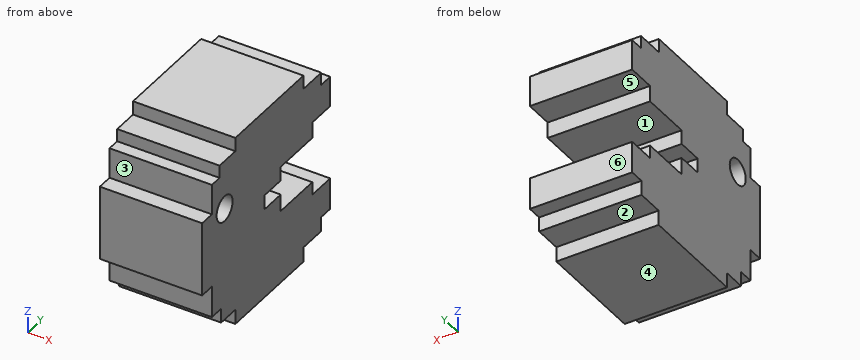
from build123d import *

# Parameters (mm, degrees)
F0_W     = 25.4
F0_H     = 25.399998
F1_DEPTH = 12.7
F3_DEPTH = 25.4
F4_R     = 1.5875
F5_DEPTH = 12.7


with BuildPart() as f1:
    # F0 (on Right) → F1 (new body)
    with BuildSketch(Plane.YZ):
        with Locations((12.7, 12.699999)):
            Rectangle(F0_W, F0_H)
    extrude(amount=F1_DEPTH)

    # F2 (on face) → F3 (cut)
    with BuildSketch(Plane.YZ.offset(12.7)):
        Polygon((0, 25.399998), (0, 16.820697), (1.931377, 16.820697), (1.931377, 20.601515), (3.452925, 20.601515), (3.452925, 22.169169), (6.588236, 22.169169), (6.588236, 23.875147), (20.09774, 23.875147), (20.09774, 22.169169), (23.624913, 22.169169), (23.624913, 20.601515), (25.4, 20.601515), (25.4, 25.399998), align=None)
        Polygon((0, 0), (6.588236, 0), (6.588236, 1.835753), (3.775678, 1.835753), (3.775678, 3.633947), (1.931377, 3.633947), (1.931377, 7.553086), (0, 7.553086), align=None)
        Polygon((20.143846, 1.835753), (20.143846, 0), (25.4, 0), (25.4, 3.633947), (23.555804, 3.633947), (23.555804, 1.835753), align=None)
        Polygon((21.849825, 7.553086), (25.4, 7.553086), (25.4, 16.820697), (21.849825, 16.820697), (21.849825, 14.838074), (15.579202, 14.838074), (15.579202, 13.085988), (12.397784, 13.085988), (12.397784, 11.287794), (15.579202, 11.287794), (15.579202, 9.166849), (21.849825, 9.166849), align=None)
    extrude(amount=-F3_DEPTH, mode=Mode.SUBTRACT)

    # F4 (on face) → F5 (cut)
    with BuildSketch(Plane.YZ.offset(12.7)):
        with Locations((4.452611, 16.06866)):
            Circle(F4_R)
    extrude(amount=-F5_DEPTH, mode=Mode.SUBTRACT)


solid = f1.part
Verification items for the finished model (mm, model axes). Face numbers are marked on the shaded views. A direction names the side the tool comes from. Coordinates: 2 decimals unless noted, no trailing zeros. Loops run counter-clockwise (first coordinate to the right, second up) from the corner with the lowest first, then second, coordinate; pieces in that order, holes last. Notation, with made-up numbers: (48, 41.25) -> (73, 41.25) arc R19 ccw to (73, 47.25) -> close; hole circle Ø8 at (7, -22.75). An arc over 180 degrees is marked (long way). Answer as a JSON object with one key per item and string values. Group by question number.
Item 1: Tool access check on the marked faces 1, 2 and 3. Record the directions out of +Z, -Z, +X, -X, +Y, -Y that give a thin tool (end or side, any length) a straight path to the whole face; none if there is none.
Item 2: Mould release check, pull along Z, two halves, no side actions. Record for the marked faces 4, 5 and 6: +Z half, -Z half, draft (parallel to the pull), parting line (faces both ways), or undercut.
Item 3: Scan lines: probe 1 along Z at (x, y) = (4.25, 23); probe 2 along Z at (x, y) = (10.75, 24); probe 3 along Y at (x, z) = (8.5, 1.5). Record each from-to range of solid material in increasing order.
Item 4: Sectioned sample at A-A on y = 18.75. Record the boundary of the cut face in (x, z).
Item 5: Sectioned sample at C-C on y = 14.5. Record the boundary of the cut face in (x, z).
Item 6: Depth check by flat-ended pin: pin 1 (2 mm diameter, centred on x = 3, z = 1, fed in from +Y); pin 2 (7 mm diameter, centred on x = 3, y = 19.5, fed in from -Z); pin 3 (1.9 mm diameter, centred on x = 5, z = 18, fed in from -Y); pin 4 (2 mm diameter, centred on x = 9.5, y = 1.5, fed in from -Z). Enter the tip coordinate at first touch or a pass-through.
Item 7: Sectioned sample at D-D on z = 10.25. Record the boundary of the cut face in (x, y).
Item 8: Sectioned sample at B-B on z = 20. Record the boundary of the cut face in (x, y).
Evaluation:
{
 "1": {"face 1": "+X, -X, +Y", "face 2": "-Z, +X, -X, +Y", "face 3": "+Z, +X, -X, -Y"},
 "2": {"face 4": "-Z half", "face 5": "undercut", "face 6": "draft"},
 "3": {"probe 1": "z = 1.84 to 7.55, 16.82 to 22.17", "probe 2": "z = 3.63 to 7.55, 16.82 to 20.6", "probe 3": "y = 6.59 to 20.14"},
 "4": {"outline": "(0, 0) -> (12.7, 0) -> (12.7, 9.17) -> (0, 9.17) -> close; (0, 14.84) -> (12.7, 14.84) -> (12.7, 23.88) -> (0, 23.88) -> close"},
 "5": {"outline": "(0, 0) -> (12.7, 0) -> (12.7, 11.29) -> (0, 11.29) -> close; (0, 13.09) -> (12.7, 13.09) -> (12.7, 23.88) -> (0, 23.88) -> close"},
 "6": {"pin 1": "stops at y = 23.56", "pin 2": "stops at z = 0", "pin 3": "stops at y = 1.93", "pin 4": "stops at z = 3.63"},
 "7": {"outline": "(0, 0) -> (12.7, 0) -> (12.7, 15.58) -> (0, 15.58) -> close"},
 "8": {"outline": "(0, 1.93) -> (12.7, 1.93) -> (12.7, 25.4) -> (0, 25.4) -> close"}
}
